The drawing under review shows one solid part. Ordinate dimensions are in mm from its lowest x, y, z. Round coordinates to 2 decimals unless told otherwise and drop trailing zeros. Write each loop counter-clockwise with the first axis right and the second up, starting at its lowest first coordinate (ties: lowest second). Pieces come first, ordered by that corner, then holes.
Item 1: Clearance check with flat-ended pins moving along their axes: pin 1 Ø2 at (x, z) = (12.5, 8.5) entering from +Y; pin 2 Ø5 at (y, z) = (7, 14) entering from +X; pin 3 Ø8 at (x, z) = (2.5, 14.5) entering from -Y; pin 4 Ø8 at (x, z) = (5, 4) entering from +Y. State where each tip first meets the part, or that it passes through.
Item 2: Add section A-A (z = 5). Give the boundary of the cut face in (x, y) (1 decimal).
Item 3: Draft analysis for pull direction Y (two halves, no side actions). For the marked faces 1 and 2, state which applies: +Y half, -Y half, draft (parallel to the pull), parting line (faces both ways), or undercut.
Item 4: Add section B-B (z = 9.75). Give the boundary of the cut face in (x, y).
Item 5: To check wall thickness, follow L1, parallel to X at y = 8, z = 2.5 (1 decimal); L2, parallel to X at y = 9.25, z = 14.25 (1 decimal); L3, parallel to X at y = 7.75, z = 23.75 (1 decimal). State the ranges of each line that lie inside material, in increasing order.
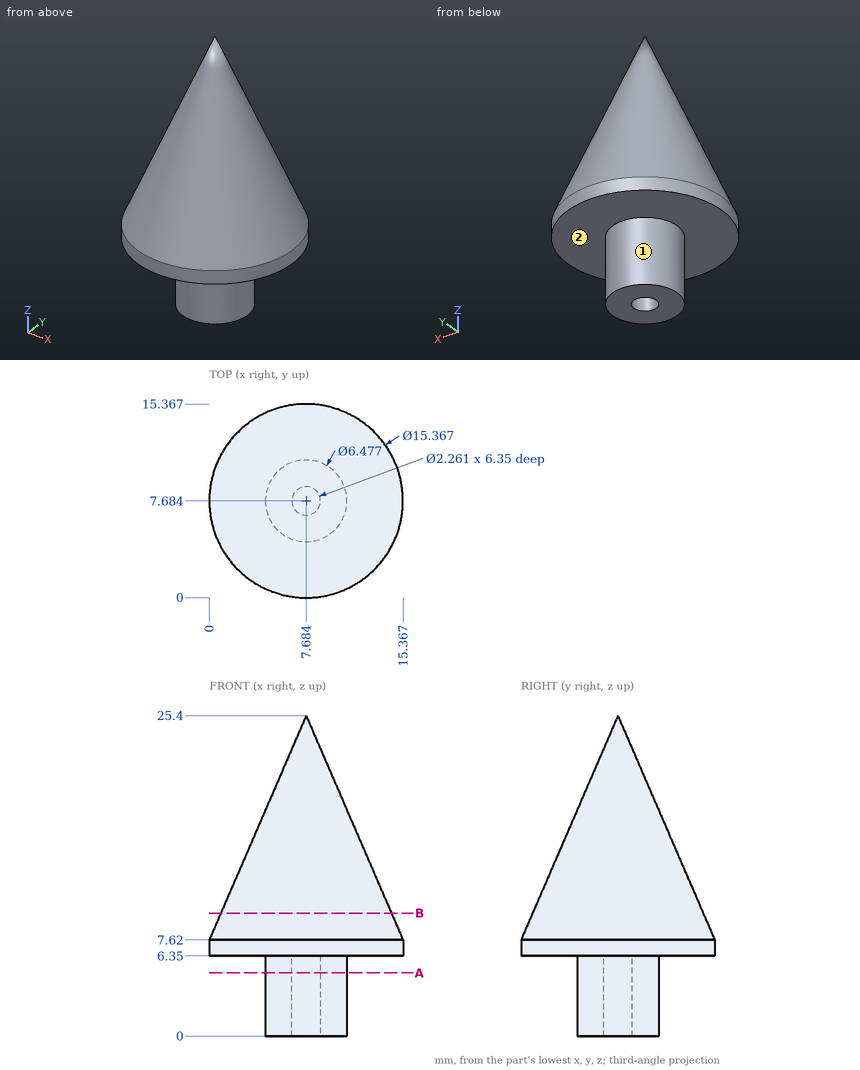
Numbers:
1. pin 1: stops at y = 14.09
1. pin 2: stops at x = 13.67
1. pin 3: stops at y = 2.24
1. pin 4: stops at y = 15.37
2. outline: circle Ø6.5 at (7.7, 7.7); hole circle Ø2.3 at (7.7, 7.7)
3. face 1: parting line
3. face 2: draft
4. outline: circle Ø13.53 at (7.68, 7.68)
5. L1: x = 4.5 to 6.6, 8.8 to 10.9
5. L2: x = 3.1 to 12.2
5. L3: x = 7 to 8.4
